```python
from build123d import *

# Parameters (mm, degrees)
VYSUNOUT_TENKOST_NN_1_DEPTH = 10
P_EV_ST_OBJEM1_START        = -10
P_EV_ST_OBJEM1_DEPTH        = 20
P_EV_ST_OBJEM1_2_DEPTH      = 20
SKICA10_W                   = 2
SKICA10_H                   = 10
ODEBRAT_VYSUNUT_M3_DEPTH    = 3.5


# Read off the part's stored shape, not the designer's step: Převést-Objem1
with BuildPart() as part:
    # Skica1 → Vysunout tenkostěnný1 (new, symmetric)
    with BuildSketch(Plane(origin=(0, 0, 0), x_dir=(0, 0, -1), z_dir=(1, 0, 0))):
        Polygon((-3.5, 10), (-3.5, 0), (2.5, 0), (2.5, 1), (-2.5, 1), (-2.5, 10), align=None)
    extrude(amount=VYSUNOUT_TENKOST_NN_1_DEPTH, both=True)

    # Převést-Objem1 outline → Převést-Objem1 (cut)
    with BuildSketch(Plane.YZ.offset(P_EV_ST_OBJEM1_START)):
        with BuildLine():
            Line((0, 3.5), (0, 1.5))
            ThreePointArc((0, 1.5), (0.585786438, 2.914213562), (2, 3.5))
            Line((2, 3.5), (0, 3.5))
        make_face()
    extrude(amount=P_EV_ST_OBJEM1_DEPTH, mode=Mode.SUBTRACT)

    # P_ev_st-Objem1 2 outline → P_ev_st-Objem1 2 (add)
    with BuildSketch(Plane.YZ.offset(P_EV_ST_OBJEM1_START)):
        with BuildLine():
            Line((1, 2.5), (1, 1.5))
            ThreePointArc((1, 1.5), (1.292893219, 2.207106781), (2, 2.5))
            Line((2, 2.5), (1, 2.5))
        make_face()
    extrude(amount=P_EV_ST_OBJEM1_2_DEPTH)

    # Skica10 → Odebrat vysunutím3 (cut)
    with BuildSketch(Plane.XY.offset(3.5)):
        with Locations((-7, 5)):
            Rectangle(SKICA10_W, SKICA10_H)
        with Locations((-2.333333333, 5)):
            Rectangle(SKICA10_W, SKICA10_H)
        with Locations((2.333333333, 5)):
            Rectangle(SKICA10_W, SKICA10_H)
        with Locations((7, 5)):
            Rectangle(SKICA10_W, SKICA10_H)
    extrude(amount=-ODEBRAT_VYSUNUT_M3_DEPTH, mode=Mode.SUBTRACT)


solid = part.part
```
Model file for the job. Use its own axes, mm. A direction names the side the tool comes from. Round coordinates to 2 decimals unless told otherwise and drop trailing zeros. Loops run counter-clockwise (first coordinate to the right, second up) from the corner with the lowest first, then second, coordinate; pieces in that order, holes last. Notation, with made-up numbers: M -18.75,-24 L 33.25,-24 A24 ccw 33.25,-6 Z; hole C -6.5,69 d7. An arc over 180 degrees is marked long. Put each result on its own line as item: value. Start each with the question number.
Item 1: Cut at C-C (x = 4.25). List the corners of the cut face in (y, z), then the cut area to 3 significant figures.
Item 2: 3-axis set-ups, long thin cutter, end or side, ignore diameter. For faces 4 (the face through (-9, 6, 2.5)), 5 (the face through (4.65, 0.57, 2.9)), 6 (the face through (7, 0.5, 0)): which of +Z, -Z, +X, -X, +Y, -Y reach the whole face in a straight line?
Item 3: Cut at A-A (z = 3.1). List the corners of the cut face in (x, y), then the cut area to 3 significant figures.
Item 4: Cut at B-B (y = 5.75). List the corners of the cut face in (x, z).
Item 5: Mould opens along X. For faces 1 (the face through (-1.333, 4, 3)), 2 (the face through (-10, 3, 3)), 3 (the face through (0, 6, 3.5)) say: released by +X, released by -X, zero draft, split by the parting line, or undercut.
Item 6: Drill centre lines: line 1 along X through (y, z) = (3, 3); line 2 along Y through (x, z) = (-3.75, 1.45); line 3 along Z through (x, y) = (0.5, 7). Where is each one in solid material? Low to high.
Item 7: Drop flat-ended pins along their axis: P1, Ø1.5, axis at x = -2, z = 0.5, coming from the +Y side; P2, Ø0.8, axis at x = -0.5, y = 7.5, coming from the -Z side; P3, Ø0.8, axis at x = -6.5, y = 0.5, coming from the +Z side; P4, Ø1.8, axis at y = 6, z = 2, coming from the +X side. Give the stop position or say it passes through.
Item 8: Cut at D-D (x = -7). List the corners of the cut face in (y, z).
Answer block:
1. outline: M 0,-2.5 L 1,-2.5 L 1,1.5 A1 cw 2,2.5 L 10,2.5 L 10,3.5 L 2,3.5 A2 ccw 0,1.5 Z
1. area: 14.4 mm2
2. face 4: -Z, +X, -X, +Y
2. face 5: +Z, +X, -X, -Y
2. face 6: +Z, +Y, -Y
3. outline: M -10,0.8 L -8,0.8 L -8,10 L -10,10 Z; M -6,0.8 L -3.33,0.8 L -3.33,10 L -6,10 Z; M -1.33,0.8 L 1.33,0.8 L 1.33,10 L -1.33,10 Z; M 3.33,0.8 L 6,0.8 L 6,10 L 3.33,10 Z; M 8,0.8 L 10,0.8 L 10,10 L 8,10 Z
3. area: 110 mm2
4. outline: M -10,2.5 L -8,2.5 L -8,3.5 L -10,3.5 Z; M -6,2.5 L -3.33,2.5 L -3.33,3.5 L -6,3.5 Z; M -1.33,2.5 L 1.33,2.5 L 1.33,3.5 L -1.33,3.5 Z; M 3.33,2.5 L 6,2.5 L 6,3.5 L 3.33,3.5 Z; M 8,2.5 L 10,2.5 L 10,3.5 L 8,3.5 Z
5. face 1: undercut
5. face 2: released by -X
5. face 3: zero draft
6. line 1: -10 to -8, -6 to -3.33, -1.33 to 1.33, 3.33 to 6, 8 to 10
6. line 2: 0 to 1
6. line 3: 2.5 to 3.5
7. P1: y = 1
7. P2: z = 2.5
7. P3: z = 0
7. P4: x = 10
8. outline: M 0,-2.5 L 1,-2.5 L 1,0 L 0,0 Z
